Solid Edge part; units mm, degrees
sketch "Sketch1" plane through (0, 0, 0) normal (0, 0, 1) x (1, 0, 0)
  line L0 (-152.4, -152.4) -> (152.4, -152.4)
  line L1 (152.4, -152.4) -> (152.4, -76.2)
  line L2 (-63.5, -76.2) -> (152.4, -76.2)
  line L3 (-63.5, -10.16) -> (-63.5, -76.2)
  line L4 (152.4, -10.16) -> (-63.5, -10.16)
  line L5 (152.4, -10.16) -> (152.4, 152.4)
  line L6 (152.4, 152.4) -> (-152.4, 152.4)
  line L7 (-152.4, 152.4) -> (-152.4, -152.4)
extrude "Protrusion1" add sketch "Sketch1" along normal blind 3.175
sketch "Sketch2" plane through (0, 0, 3.175) normal (0, 0, 1) x (0, 1, 0)
  line L0 (-79.375, -152.4) -> (-76.2, -152.4)
  line L1 (-76.2, -152.4) -> (-76.2, 63.5)
  line L2 (-76.2, 63.5) -> (-79.375, 63.5)
  line L3 (-79.375, 63.5) -> (-79.375, -152.4)
  line L4 (-10.16, -152.4) -> (-6.985, -152.4)
  line L5 (-6.985, -152.4) -> (-6.985, 63.5)
  line L6 (-6.985, 63.5) -> (-10.16, 63.5)
  line L7 (-10.16, 63.5) -> (-10.16, -152.4)
  dimension "D1" = 76.2
  dimension "D2" = 6.985
extrude "ExtrudedProtrusion_2" add sketch "Sketch2" along normal blind 63.5
sketch "Sketch3" plane through (0, 0, 3.175) normal (0, 0, 1) x (0, 1, 0)
  line L0 (139.7, -76.2) -> (114.3, -76.2)
  line L1 (114.3, -76.2) -> (114.3, 76.2)
  line L2 (114.3, 76.2) -> (139.7, 76.2)
  line L3 (139.7, 76.2) -> (139.7, -76.2)
  line L4 (-139.7, -76.2) -> (-114.3, -76.2)
  line L5 (-114.3, -76.2) -> (-114.3, 76.2)
  line L6 (-114.3, 76.2) -> (-139.7, 76.2)
  line L7 (-139.7, 76.2) -> (-139.7, -76.2)
  dimension "D1" = 114.3
  dimension "D2" = 114.3
  dimension "D3" = 114.3
  dimension "D4" = 114.3
extrude "Cutout1" cut sketch "Sketch3" against normal through all
sketch "Sketch4" plane through (44.45, -76.2, 33.3375) normal (0, 1, 0) x (-1, 0, 0)
  circle A0 centre (-48.26, -23.8125) radius 0.7938
  circle A1 centre (101.6, -23.8125) radius 0.7938
  circle A2 centre (-95.25, -23.8125) radius 0.7938
extrude "ExtrudedProtrusion_3" add sketch "Sketch4" along normal blind 66.04
sketch "Sketch5" plane through (0, 0, 3.175) normal (0, 0, 1) x (0, 1, 0)
  line L0 (-104.775, -152.4) -> (-79.375, -152.4)
  line L1 (-79.375, -152.4) -> (-79.375, -101.6)
  line L2 (-79.375, -101.6) -> (-104.775, -101.6)
  line L3 (-104.775, -101.6) -> (-104.775, -152.4)
  line L4 (-6.985, -152.4) -> (18.415, -152.4)
  line L5 (18.415, -152.4) -> (18.415, -101.6)
  line L6 (18.415, -101.6) -> (-6.985, -101.6)
  line L7 (-6.985, -101.6) -> (-6.985, -152.4)
  dimension "D1" = 79.375
  dimension "D2" = 104.775
  dimension "D3" = 18.415
  dimension "D4" = 18.415
extrude "ExtrudedProtrusion_4" add sketch "Sketch5" along normal blind 355.6
sketch "Sketch6" plane through (120.65, 61.595, 180.975) normal (0, 1, 0) x (0, 0, -1)
  circle A0 centre (-152.4, 0) radius 6.35
extrude "Cutout2" cut sketch "Sketch6" against normal through all
Check sheet for the modelled part. Datum: model origin and axes. Units: mm. A direction names the side the tool comes from. Coordinates: 2 decimals unless noted, no trailing zeros. Order: outer loops, then holes, each group sorted by start corner. A loop starts at its lowest first (then second) coordinate and runs counter-clockwise, first axis right, second up. Notation, with made-up numbers: M 78,4 L 133,4 A17 cw 133,25 Z; hole C -13,52.25 d10. An arc over 180 degrees is marked long. One line per question, with ' | ' between items. Start each with the question number.
Item 1: Mould release check, pull along Z, two halves, no side actions. Record for faces 5 (the flat face through (18, -79.375, 34)), 6 (the cylindrical face through (120.37, 5.89, 339.72)), 7 (the flat face through (-2, 2, 0)), 8 (the cylindrical face through (120.37, -91.9, 339.72)): pulls with the +Z half, pulls with the -Z half, needs draft (parallel to the pull), parting line crosses it, or undercut.
Item 2: Sectioned sample at B-B on x = -19. Record the cut outline in (y, z) (3 decimals).
Item 3: Sectioned sample at D-D on z = 85. Record the cut outline in (x, y) (3 decimals), and give its area (3 significant figures).
Item 4: Material ranges on line 1 (Z direction, x = 120.65, y = 3.75) (3 decimals); line 2 (Y direction, x = 114, z = 105.5) (3 decimals); line 3 (Y direction, x = -34.5, z = 18.5) (3 decimals), recorded low to high.
Item 5: Sectioned sample at A-A on z = 47.5. Record the cut outline in (x, y) (3 decimals).
Item 6: Access from +Z, -Z, +X, -X, +Y, -Y to the whole of each face (thin tool, end or side, straight path). Record for faces 1 (the flat face through (-2, 2, 3.175)), 2 (the flat face through (101.6, -92, 178)), 3 (the flat face through (127, -104.775, 178)), 4 (the flat face through (127, 18.415, 178)).
Item 7: Sectioned sample at C-C on y = -122. Record the cut outline in (x, z) (3 decimals), and give its area (3 significant figures).
Item 8: Gauge pin test, flat ends, axial feed: P1, Ø6, axis at x = 40.5, y = -107, coming from the +Z side (3 decimals); P2, Ø20.5, axis at x = 120.65, z = 333.375, coming from the +Y side (3 decimals); P3, Ø20, axis at x = 60.5, z = 40, coming from the -Y side (3 decimals). Record the tip position at first contact, or that the pin passes through.
Answer below:
1) face 5: needs draft | face 6: undercut | face 7: pulls with the -Z half | face 8: undercut
2) outline: M -152.4,0 L -139.7,0 L -139.7,3.175 L -152.4,3.175 Z; M -114.3,0 L -76.2,0 L -76.2,66.675 L -79.375,66.675 L -79.375,3.175 L -114.3,3.175 Z; M -10.16,0 L 114.3,0 L 114.3,3.175 L -6.985,3.175 L -6.985,66.675 L -10.16,66.675 Z; M 139.7,0 L 152.4,0 L 152.4,3.175 L 139.7,3.175 Z
3) outline: M 101.6,-104.775 L 152.4,-104.775 L 152.4,-79.375 L 101.6,-79.375 Z; M 101.6,-6.985 L 152.4,-6.985 L 152.4,18.415 L 101.6,18.415 Z | area: 2,580 mm^2
4) line 1: z = 0 to 327.025, 339.725 to 358.775 | line 2: y = -104.775 to -79.375, -6.985 to 18.415 | line 3: y = -79.375 to -76.2, -10.16 to -6.985
5) outline: M -63.5,-79.375 L 101.6,-79.375 L 101.6,-104.775 L 152.4,-104.775 L 152.4,-76.2 L -63.5,-76.2 Z; M -63.5,-10.16 L 152.4,-10.16 L 152.4,18.415 L 101.6,18.415 L 101.6,-6.985 L -63.5,-6.985 Z
6) face 1: +Z, -X | face 2: +Z, -X, -Y | face 3: +Z, +X, -X, -Y | face 4: +Z, +X, -X, +Y
7) outline: M -152.4,0 L -76.2,0 L -76.2,3.175 L -152.4,3.175 Z; M 76.2,0 L 152.4,0 L 152.4,3.175 L 76.2,3.175 Z | area: 484 mm^2
8) P1: stops at z = 3.175 | P2: stops at y = 18.415 | P3: stops at y = -79.375
